```python
from build123d import *

# Parameters (mm, degrees)
F_0060_CYLINDER_SKETCH_R    = 3.25
F_0060_CYLINDER_DEPTH       = 2.5
F_0061_FILLET_R             = 0.625
F_0062_EXTRUDE_DEPTH        = 1.385
F_0062_EXTRUDE_ROTATE_ANGLE = 120
F_0065_CYLINDER_SKETCH_R    = 1.2
F_0065_CYLINDER_DEPTH       = 15.7
F_0066_CONE_ROTATE_ANGLE    = 90


with BuildPart() as part:
    # 0060_cylinder_Sketch → 0060_cylinder (new body)
    with BuildSketch(Plane.XY):
        Circle(F_0060_CYLINDER_SKETCH_R)
    extrude(amount=F_0060_CYLINDER_DEPTH)

    # 0061_fillet
    f_0061_fillet_edges = [part.edges().sort_by_distance(p)[0] for p in [
        (-3.25, 0, 2.5),
    ]]
    fillet(f_0061_fillet_edges, radius=F_0061_FILLET_R)


with BuildPart() as body_2:
    # 0062_extrude_Sketch → 0062_extrude (new body)
    with BuildSketch(Plane.XY):
        Polygon((0, 0), (1.154700538, 0), (1.732050808, 1), (1.154700538, 2), (0, 2), (-0.577350269, 1), align=None)
    extrude(amount=F_0062_EXTRUDE_DEPTH)


with BuildPart() as body_2_1:
    # 0062_extrude_Rotate: read off the stored shape, not the designer's step
    # 0062_extrude_Rotate: moved
    add(body_2.part.rotate(Axis((0, 0, 0), (0, 0, 1)), F_0062_EXTRUDE_ROTATE_ANGLE))


with BuildPart() as body_2_2:
    # 0062_extrude_Translate: moved
    add(body_2_1.part.moved(Location((1.154700538, 0, 1.125))))


with BuildPart() as part_1:
    add(part.part)

    # 0064_sub: cut body 2
    add(body_2_2.part, mode=Mode.SUBTRACT)


with BuildPart() as body_2_2_1:
    # 0065_cylinder_Sketch → 0065_cylinder (new body)
    with BuildSketch(Plane.XY):
        Circle(F_0065_CYLINDER_SKETCH_R)
    extrude(amount=F_0065_CYLINDER_DEPTH)


with BuildPart() as body_2_2_2:
    # 0065_cylinder_Translate: moved
    add(body_2_2_1.part.moved(Location((0, 0, -15.7))))


with BuildPart() as body_3:
    # 0066_cone_Sketch → 0066_cone (revolve)
    with BuildSketch(Plane.XY, mode=Mode.PRIVATE) as f_0066_cone_sk:
        Polygon((0, 0), (1.2, 0), (0.9, 0.3), (0, 0.3), align=None)
    revolve(f_0066_cone_sk.sketch.rotate(Axis((0, -100, 0), (0, 1, 0)), 90), axis=Axis((0, -100, 0), (0, 1, 0)))


with BuildPart() as body_3_1:
    # 0066_cone_Rotate: moved
    add(body_3.part.rotate(Axis((0, 0, 0), (1, 0, 0)), F_0066_CONE_ROTATE_ANGLE))


with BuildPart() as body_3_2:
    # 0066_cone_Translate: moved
    add(body_3_1.part.moved(Location((0, 0, -16))))


with BuildPart() as body_2_2_3:
    add(body_2_2_2.part)

    # 0068_add: union body 3
    add(body_3_2.part)


with BuildPart() as part_2:
    add(part_1.part)

    # 0069_add: union body 2 2
    add(body_2_2_3.part)


solid = part_2.part
```
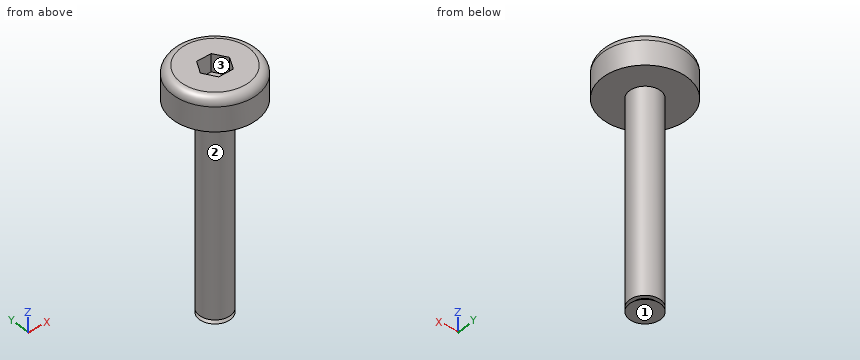
Check sheet for the modelled part. Datum: model origin and axes. Units: mm. Face numbers are marked on the shaded views. A direction names the side the tool comes from. Coordinates: 2 decimals unless noted, no trailing zeros. Order: outer loops, then holes, each group sorted by start corner. A loop starts at its lowest first (then second) coordinate and runs counter-clockwise, first axis right, second up. Notation, with made-up numbers: (7, -10.75) -> (37, -10.75) arc R7 ccw to (37, -1.75) -> close; hole circle Ø3 at (81, -36.75). An arc over 180 degrees is marked (long way). Write each question's results on one line, items separated by ' | '. Start each with the question number.
1) Depth check by flat-ended pin: pin 1 (2 mm diameter, centred on x = -2, y = -2, fed in from -Z); pin 2 (1.6 mm diameter, centred on x = 0, y = 0, fed in from +Z) (3 decimals); pin 3 (3 mm diameter, centred on x = -1, y = -1, fed in from -Z); pin 4 (1.5 mm diameter, centred on y = 0.5, z = -4.5, fed in from -X). Enter the tip coordinate at first touch or a pass-through.
2) Set-up check for the marked faces 1, 2 and 3: record each of +Z, -Z, +X, -X, +Y, -Y from which the full face is reachable in a straight line by a thin tool's end or side.
3) Material ranges on line 1 along Z through (x, y) = (0.75, 0) (3 decimals); line 2 along Z through (x, y) = (1.5, 0.25); line 3 along X through (y, z) = (-1, -9.25), recorded low to high.
4) Section check A-A (x = 0). Enter the section's corners in (y, z) (3 decimals).
5) Section check B-B (z = -6.5). Enter the section's corners in (x, y), and give its area (3 significant figures).
Checked values:
1) pin 1: z = 0 | pin 2: z = 1.125 | pin 3: z = -16 | pin 4: x = -1.2
2) face 1: -Z, +X, -X, +Y, -Y | face 2: -Z | face 3: +Z
3) line 1: -16 to 1.125 | line 2: 0 to 2.5 | line 3: -0.66 to 0.66
4) outline: (-3.25, 0) -> (-1.2, 0) -> (-1.2, -15.7) -> (-0.9, -15.7) -> (-1.2, -16) -> (1.2, -16) -> (0.9, -15.7) -> (1.2, -15.7) -> (1.2, 0) -> (3.25, 0) -> (3.25, 1.875) arc R0.625 ccw to (2.625, 2.5) -> (1, 2.5) -> (1, 1.125) -> (-1, 1.125) -> (-1, 2.5) -> (-2.625, 2.5) arc R0.625 ccw to (-3.25, 1.875) -> close
5) outline: circle Ø2.4 at (0, 0) | area: 4.52 mm²
